from build123d import *

# Parameters (mm, degrees)
F0_W    = 1.8
F0_H    = 0.8
F2_SIZE = 0.5


with BuildPart() as f1:
    # F0 (on Front) → F1 (revolve)
    with BuildSketch(Plane.XZ):
        with Locations((-10.141778, 7.541778)):
            Rectangle(F0_W, F0_H)
        Polygon((0, -2), (0, 0), (-7.141778, 7.141778), (-9.241778, 7.141778), (-11.041778, 7.141778), (-12.141778, 7.141778), (-12.141778, -2), align=None)
    revolve(axis=Axis((15, 0, 2.570889), (0, 0, 1)))

    # F2
    f2_edges = [f1.edges().sort_by_distance(p)[0] for p in [
        (30, 0, 0),
    ]]
    chamfer(f2_edges, length=F2_SIZE)


solid = f1.part
Geometry check sheet. Reference: the model listing, model coordinates, mm. A direction names the side the tool comes from. Give positions to 0.01 mm unless a question says otherwise; leave off trailing zeros. Order: outer loops, then holes, each group sorted by start corner. A loop starts at its lowest first (then second) coordinate and runs counter-clockwise, first axis right, second up. Notation, with made-up numbers: (35, 25) - (56, 25) arc R26 cw to (56, 49) - close; hole circle Ø1 at (-14, 16). An arc over 180 degrees is marked (long way). Use one line per item in the form item = value.
1) Draft check along Y on faces 1 (the face through (34.194, -17.6, 7.547)), 2 (the face through (3, 12, -2)), 3 (the face through (-0.05, -4.74, 0.78)). Enter one of: released by +Y, released by -Y, zero draft, split by the parting line, or undercut.
Working result:
face_1 = split by the parting line
face_2 = zero draft
face_3 = undercut
2) Material ranges on probe 1 along X at (y, z) = (0, -1.3); probe 2 along Y at (x, z) = (15, 7.7); probe 3 along X at (y, z) = (0, 7.7), recorded low to high. Write a range as from..to.
Working result:
probe_1 = -12.14..0, 30..42.14
probe_2 = -26.04..-24.24, 24.24..26.04
probe_3 = -11.04..-9.24, 39.24..41.04
3) Depth check by flat-ended pin: pin 1 Ø4 at (y, z) = (12, 3) entering from -X; pin 2 Ø2 at (x, y) = (2.5, 0) entering from -Z; pin 3 Ø5 at (y, z) = (-8, 3) entering from -X; pin 4 Ø6 at (x, y) = (8, 15.5) entering from +Z. Enter the tip coordinate at first touch or a pass-through.
Working result:
pin_1 = -10.23
pin_2 = through
pin_3 = -11.58
pin_4 = 5.01
4) Access from +Z, -Z, +X, -X, +Y, -Y to the whole of each face (thin tool, end or side, straight path). Record for faces 4 (the face through (34.2, 14.8, 7.5)), 5 (the face through (-4.2, 15.3, 7.942)).
Working result:
face_4 = +Z
face_5 = +Z, +X, -X, +Y, -Y
5) Sectioned sample at A-A (z = 1.25). Record the boundary of the cut face in (x, y).
Working result:
outline = circle Ø54.28 at (15, 0); hole circle Ø32.5 at (15, 0)
